The listing builds one solid part. Answer for the finished solid, in the listing's coordinates (mm). Face numbers are marked on the shaded views. A direction names the side the tool comes from. Round coordinates to 2 decimals unless told otherwise and drop trailing zeros. Loops run counter-clockwise (first coordinate to the right, second up) from the corner with the lowest first, then second, coordinate; pieces in that order, holes last. Notation, with made-up numbers: (-5, 34) - (48, 34) arc R27 cw to (48, 56) - close; hole circle Ø5 at (9, 14). An arc over 180 degrees is marked (long way). One line per item, written item: value.
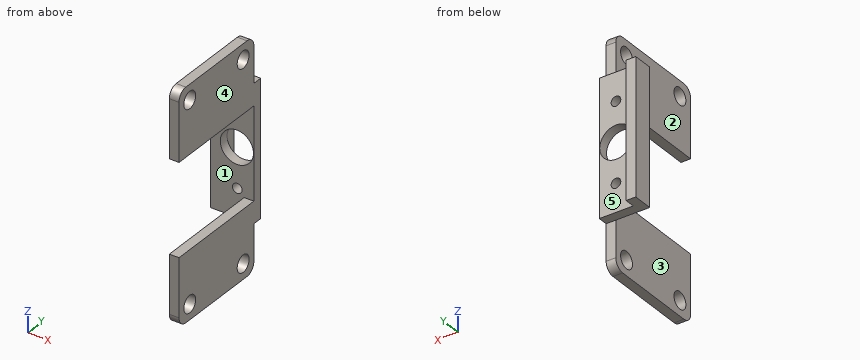
```python
from build123d import *

# Parameters (mm, degrees)
BOSS_EXTRUDE3_DEPTH = 28
SKETCH4_R           = 3.43
SKETCH4_R_2         = 1
CUT_EXTRUDE1_DEPTH  = 2
SKETCH6_W           = 2
SKETCH6_H           = 22
BOSS_EXTRUDE4_DEPTH = 9.5
SKETCH7_W           = 2
SKETCH7_H           = 22
BOSS_EXTRUDE5_DEPTH = 9.5
FILLET1_R           = 2
FILLET2_R           = 2
FILLET3_R           = 2
CUT_EXTRUDE2_REACH  = 4
SKETCH8_R           = 1.75
CUT_EXTRUDE3_REACH  = 11
SKETCH9_W           = 19
SKETCH9_H           = 22


with BuildPart() as part:
    # Sketch3 → Boss-Extrude3 (new body)
    with BuildSketch(Plane.XY):
        Polygon((-16.953175304, 6.6875), (-14.953175304, 6.6875), (-14.953175304, 4.5875), (-7.953175304, 4.5875), (-7.953175304, -19.4125), (-9.953175304, -19.4125), (-9.953175304, 2.5875), (-16.953175304, 2.5875), align=None)
    extrude(amount=BOSS_EXTRUDE3_DEPTH)

    # Sketch4 → Cut-Extrude1 (cut)
    with BuildSketch(Plane(origin=(0, 4.5875, 0), x_dir=(1, 0, 0), z_dir=(0, 1, 0))):
        with Locations((-11.458423587, -14)):
            Circle(SKETCH4_R)
        with Locations((-11.383175304, -5.822)):
            Circle(SKETCH4_R_2)
        with Locations((-11.383175304, -22.177653801)):
            Circle(SKETCH4_R_2)
    extrude(amount=-CUT_EXTRUDE1_DEPTH, mode=Mode.SUBTRACT)

    # Sketch6 → Boss-Extrude4 (add)
    with BuildSketch(Plane(origin=(0, 0, 0), x_dir=(-1, 0, 0), z_dir=(0, 0, -1))):
        with Locations((8.953175304, -8.4125)):
            Rectangle(SKETCH6_W, SKETCH6_H)
    extrude(amount=BOSS_EXTRUDE4_DEPTH)

    # Sketch7 → Boss-Extrude5 (add)
    with BuildSketch(Plane.XY.offset(28)):
        with Locations((-8.953175304, -8.4125)):
            Rectangle(SKETCH7_W, SKETCH7_H)
    extrude(amount=BOSS_EXTRUDE5_DEPTH)

    # Fillet1
    fillet1_edges = [part.edges().sort_by_distance(p)[0] for p in [
        (-8.953175304, 2.5875, 37.5),
    ]]
    fillet(fillet1_edges, radius=FILLET1_R)

    # Fillet2
    fillet2_edges = [part.edges().sort_by_distance(p)[0] for p in [
        (-8.953175304, 2.5875, -9.5),
    ]]
    fillet(fillet2_edges, radius=FILLET2_R)

    # Fillet3
    fillet3_edges = [part.edges().sort_by_distance(p)[0] for p in [
        (-8.953175304, -19.4125, -9.5),
        (-8.953175304, -19.4125, 37.5),
    ]]
    fillet(fillet3_edges, radius=FILLET3_R)

    # Sketch8 → Cut-Extrude2 (cut, up to next)
    with BuildSketch(Plane.ZY.offset(9.953175304), mode=Mode.PRIVATE) as cut_extrude2_sk1:
        with Locations((34.35, -0.5625)):
            Circle(SKETCH8_R)
    cut_extrude2_tool1 = extrude(cut_extrude2_sk1.sketch, amount=-CUT_EXTRUDE2_REACH, mode=Mode.PRIVATE) & part.part
    add(cut_extrude2_tool1.solids().sort_by_distance((-9.953175, -0.5625, 34.35))[0], mode=Mode.SUBTRACT)
    # Sketch8 → Cut-Extrude2 (cut, up to next)
    with BuildSketch(Plane.ZY.offset(9.953175304), mode=Mode.PRIVATE) as cut_extrude2_sk2:
        with Locations((-6.35, -0.5625)):
            Circle(SKETCH8_R)
    cut_extrude2_tool2 = extrude(cut_extrude2_sk2.sketch, amount=-CUT_EXTRUDE2_REACH, mode=Mode.PRIVATE) & part.part
    add(cut_extrude2_tool2.solids().sort_by_distance((-9.953175, -0.5625, -6.35))[0], mode=Mode.SUBTRACT)
    # Sketch8 → Cut-Extrude2 (cut, up to next)
    with BuildSketch(Plane.ZY.offset(9.953175304), mode=Mode.PRIVATE) as cut_extrude2_sk3:
        with Locations((-6.35, -16.2625)):
            Circle(SKETCH8_R)
    cut_extrude2_tool3 = extrude(cut_extrude2_sk3.sketch, amount=-CUT_EXTRUDE2_REACH, mode=Mode.PRIVATE) & part.part
    add(cut_extrude2_tool3.solids().sort_by_distance((-9.953175, -16.2625, -6.35))[0], mode=Mode.SUBTRACT)
    # Sketch8 → Cut-Extrude2 (cut, up to next)
    with BuildSketch(Plane.ZY.offset(9.953175304), mode=Mode.PRIVATE) as cut_extrude2_sk4:
        with Locations((34.35, -16.2625)):
            Circle(SKETCH8_R)
    cut_extrude2_tool4 = extrude(cut_extrude2_sk4.sketch, amount=-CUT_EXTRUDE2_REACH, mode=Mode.PRIVATE) & part.part
    add(cut_extrude2_tool4.solids().sort_by_distance((-9.953175, -16.2625, 34.35))[0], mode=Mode.SUBTRACT)

    # Sketch9 → Cut-Extrude3 (cut, up to next)
    with BuildSketch(Plane(origin=(-7.953175304, 0, 0), x_dir=(0, 0, -1), z_dir=(1, 0, 0)), mode=Mode.PRIVATE) as cut_extrude3_sk1:
        with Locations((-14, -8.4125)):
            Rectangle(SKETCH9_W, SKETCH9_H)
    cut_extrude3_tool1 = extrude(cut_extrude3_sk1.sketch, amount=-CUT_EXTRUDE3_REACH, mode=Mode.PRIVATE) & part.part
    add(cut_extrude3_tool1.solids().sort_by_distance((-7.953175, -8.4125, 14))[0], mode=Mode.SUBTRACT)


solid = part.part
```
1) A cutting plane is placed at A-A on z = 34.35. Give the vertices of the cut face in (x, y).
Final values:
outline: (-9.95, -19.41) - (-7.95, -19.41) - (-7.95, -18.01) - (-9.95, -18.01) - close; (-9.95, -14.51) - (-7.95, -14.51) - (-7.95, -2.31) - (-9.95, -2.31) - close; (-9.95, 1.19) - (-7.95, 1.19) - (-7.95, 2.59) - (-9.95, 2.59) - close
2) A cutting plane is placed at C-C on z = 14. Give the vertices of the cut face in (x, y), and give its area (3 significant figures).
Final values:
outline: (-16.95, 2.59) - (-14.89, 2.59) - (-14.89, 4.59) - (-14.95, 4.59) - (-14.95, 6.69) - (-16.95, 6.69) - close; (-8.03, 2.59) - (-7.95, 2.59) - (-7.95, 4.59) - (-8.03, 4.59) - close
area: 8.48 mm2
3) For a pull along Z with two mould halves and no side action, classify the marked faces 1 and 2 as released by +Z, released by -Z, zero draft, split by the parting line, or undercut.
Final values:
face 1: undercut
face 2: zero draft
4) A cutting plane is placed at B-B on y = -7. Give the vertices of the cut face in (x, z).
Final values:
outline: (-9.95, -9.5) - (-7.95, -9.5) - (-7.95, 4.5) - (-9.95, 4.5) - close; (-9.95, 23.5) - (-7.95, 23.5) - (-7.95, 37.5) - (-9.95, 37.5) - close
5) Each of these flat-tipped pins is pushed along its axis until it touches: pin 1 Ø1.6 at (x, z) = (-9, -3.5) entering from +Y; pin 2 Ø4 at (y, z) = (-11, 32) entering from -X; pin 3 Ø3 at (y, z) = (-0.56, 34.35) entering from -X; pin 4 Ø1 at (x, y) = (-14, 2.5) entering from -Z. Where does it stop, or does it pass through?
Final values:
pin 1: y = 2.59
pin 2: x = -9.95
pin 3: through
pin 4: z = 0
6) Consider L1, parallel to Y at x = -8.65, z = -6.35; L2, parallel to Z at x = -8.75, y = -10.5; L3, parallel to Y at x = -9.75, z = 17.5. Determine where each line is inside the solid, lowest interval first.
Final values:
L1: -19.41 to -18.01, -14.51 to -2.31, 1.19 to 2.59
L2: -9.5 to 4.5, 23.5 to 37.5
L3: 2.59 to 4.59
7) A cutting plane is placed at D-D on x = -11.5. Give the vertices of the cut face in (y, z).
Final values:
outline: (2.59, 0) - (4.59, 0) - (4.59, 4.83) - (2.59, 4.83) - close; (2.59, 6.82) - (4.59, 6.82) - (4.59, 10.57) - (2.59, 10.57) - close; (2.59, 17.43) - (4.59, 17.43) - (4.59, 21.18) - (2.59, 21.18) - close; (2.59, 23.17) - (4.59, 23.17) - (4.59, 28) - (2.59, 28) - close
8) For the marked faces 3, 4 and 5, determine the directions among +Z, -Z, +X, -X, +Y, -Y from which every point of the face is accessible in a straight line to the end or side of a thin tool.
Final values:
face 3: +Z, -Z, -X, -Y
face 4: +Z, -Z, +X, +Y, -Y
face 5: +Z, -Z, +X, +Y
